Autodesk Fusion 360 part; units mm, degrees
sketch "Sketch1" plane through (0, 0, 0) normal (0, 0, 1) x (1, 0, 0)
  circle A0 centre (0, 0) radius 10
  dimension "d1" = 20
extrude "Extrude1" add sketch "Sketch1" along normal blind 5
sketch "Sketch2" plane through (0, 0, 5) normal (0, 0, 1) x (-1, 0, 0)
  circle A0 centre (0, 0) radius 10
  line L0 (-3, -3) -> (-3, -9.5394)
  line L1 (3, 3) -> (3, 9.5394)
  line L2 (-3, 3) -> (-3, 9.5394)
  line L3 (3, -3) -> (3, -9.5394)
  line L4 (-3, 3) -> (-9.5394, 3)
  line L5 (3, 3) -> (9.5394, 3)
  line L6 (3, -3) -> (9.5394, -3)
  line L7 (-3, -3) -> (-9.5394, -3)
extrude "Extrude2" add sketch "Sketch2" along normal blind 194.9 contours A0 L0 L1 L2 L3 L4 L5 L6 L7
sketch "Sketch3" plane through (0, 0, 0) normal (0, 0, -1) x (1, 0, 0)
  circle A0 centre (0, 0) radius 10
  circle A1 centre (0, 0) radius 2.5
  dimension "d14" = 5
extrude "Extrude3" cut sketch "Sketch3" against normal blind 17 contours A1
extrude "Extrude4" add 4 faces at (5.7029, 5.7029, 5) (-5.7029, 5.7029, 5) (5.7029, -5.7029, 5) (-5.7029, -5.7029, 5) along direction (0, 0, 1) blind 175
equation "d12 = 196 mm - 5 mm + 3.9 mm"
equation "d17 = 195.00 mm - 20 mm"
Part model, mm, in its own coordinate system. A direction names the side the tool comes from. Coordinates: 2 decimals unless noted, no trailing zeros. Order: outer loops, then holes, each group sorted by start corner. A loop starts at its lowest first (then second) coordinate and runs counter-clockwise, first axis right, second up. Notation, with made-up numbers: M 16.5,75.25 L 66.5,75.25 A14 cw 66.5,102.25 Z; hole C -7.5,66.25 d7. An arc over 180 degrees is marked long. One line per question, with ' | ' between items.
Q1. Drill centre lines: line 1 (Y direction, x = 0, z = 11.25); line 2 (Z direction, x = -5.5, y = 6.25). Where is each one in solid material? Low to high.
A:
line 1: y = -10 to -2.5, 2.5 to 10 | line 2: z = 0 to 180
Q2. Slice it at A-A (x = 0). Give the cut face in (y, z).
A:
outline: M -10,0 L -2.5,0 L -2.5,17 L 2.5,17 L 2.5,0 L 10,0 L 10,199.9 L -10,199.9 Z
Q3. Slice it at B-B (y = 5). Give the cut face in (x, z), and give its area (3 significant figures).
A:
outline: M -8.66,0 L 8.66,0 L 8.66,180 L 3,180 L 3,199.9 L -3,199.9 L -3,180 L -8.66,180 Z | area: 3,240 mm^2
Q4. Two-plate mould, pull along X, no slides. Class faces 1 (the face through (0, 0, 17)), 2 (the face through (-3, 6, 190)), 3 (the face through (-6, -3, 190)): +X half, -X half, draft (parallel to the pull), parting line (faces both ways), or undercut.
A:
face 1: undercut | face 2: -X half | face 3: draft
Q5. 3-axis set-ups, long thin cutter, end or side, ignore diameter. For faces 4 (the face through (5, -5, 180)), 5 (the face through (5, 6, 180)), 6 (the face through (-6, 6, 180)), 7 (the face through (-3, -6, 190)): which of +Z, -Z, +X, -X, +Y, -Y reach the whole face in a straight line?
A:
face 4: +Z, +X, -Y | face 5: +Z, +X, +Y | face 6: +Z, -X, +Y | face 7: +Z, -X, -Y
Q6. Pin check, flat tips, straight feed: P1, Ø2, axis at x = -7.5, y = -6.5, coming from the +Z side; P2, Ø7, axis at y = -8, z = 191.5, coming from the -X side; P3, Ø2, axis at x = -6.5, z = 187.5, coming from the +Y side. Stop position of each tip, or through.
A:
P1: stops at z = 180 | P2: stops at x = -3 | P3: stops at y = 3
